```python
from build123d import *

# Parameters (mm, degrees)
SKETCH1_R               = 20
SKETCH1_R_2             = 5
BOSS_EXTRUDE1_DEPTH     = 166
ENL_V_START             = -142.6
ESQUISSE3_R             = 20
ESQUISSE3_R_2           = 17.5
ENL_V_MAT_EXTRU_1_DEPTH = 2.4
ENL_V_START_2           = -32.2
ESQUISSE4_R             = 20
ESQUISSE4_R_2           = 17.5
ENL_V_MAT_EXTRU_2_DEPTH = 2.4
BOSS_EXTRU_1_START      = -22.8
BOSS_EXTRU_1_DEPTH      = 12.6
ESQUISSE6_R             = 20
ESQUISSE6_R_2           = 5
BOSS_EXTRU_2_DEPTH      = 110
BOSS_EXTRU_3_START      = -132.8
ESQUISSE7_R             = 40
BOSS_EXTRU_3_DEPTH      = 6
BOSS_EXTRU_4_START      = -30.2
ESQUISSE8_R             = 30
BOSS_EXTRU_4_DEPTH      = 10
CONG_3_R                = 19
ECHELLE1_SCALE          = 0.25


with BuildPart() as part:
    # Sketch1 → Boss-Extrude1 (new body)
    with BuildSketch(Plane.XY):
        Circle(SKETCH1_R)
        Circle(SKETCH1_R_2, mode=Mode.SUBTRACT)
    extrude(amount=BOSS_EXTRUDE1_DEPTH)

    # Esquisse3 → Enlèv. mat.-Extru.1 (cut)
    with BuildSketch(Plane.XY.offset(166).offset(ENL_V_START)):
        Circle(ESQUISSE3_R)
        Circle(ESQUISSE3_R_2, mode=Mode.SUBTRACT)
    extrude(amount=ENL_V_MAT_EXTRU_1_DEPTH, mode=Mode.SUBTRACT)

    # Esquisse4 → Enlèv. mat.-Extru.2 (cut)
    with BuildSketch(Plane.XY.offset(166).offset(ENL_V_START_2)):
        Circle(ESQUISSE4_R)
        Circle(ESQUISSE4_R_2, mode=Mode.SUBTRACT)
    extrude(amount=ENL_V_MAT_EXTRU_2_DEPTH, mode=Mode.SUBTRACT)

    # Esquisse5 → Boss.-Extru.1 (add)
    with BuildSketch(Plane.XY.offset(166).offset(BOSS_EXTRU_1_START)):
        with BuildLine():
            Line((-19.364916731, 5), (-26.364916731, 5))
            ThreePointArc((-26.364916731, 5), (-31.364916731, 0), (-26.364916731, -5))
            Line((-26.364916731, -5), (-19.364916731, -5))
            ThreePointArc((-19.364916731, -5), (-20, 0), (-19.364916731, 5))
        make_face()
        with BuildLine():
            Line((19.364916731, -5), (26.364916731, -5))
            ThreePointArc((26.364916731, -5), (31.364916731, 0), (26.364916731, 5))
            Line((26.364916731, 5), (19.364916731, 5))
            ThreePointArc((19.364916731, 5), (20, 0), (19.364916731, -5))
        make_face()
    extrude(amount=BOSS_EXTRU_1_DEPTH)

    # Esquisse6 → Boss.-Extru.2 (add)
    with BuildSketch(Plane.XY.offset(166)):
        Circle(ESQUISSE6_R)
        Circle(ESQUISSE6_R_2, mode=Mode.SUBTRACT)
    extrude(amount=BOSS_EXTRU_2_DEPTH)

    # Esquisse7 → Boss.-Extru.3 (add)
    with BuildSketch(Plane.XY.offset(276).offset(BOSS_EXTRU_3_START)):
        Circle(ESQUISSE7_R)
    extrude(amount=-BOSS_EXTRU_3_DEPTH)

    # Esquisse8 → Boss.-Extru.4 (add)
    with BuildSketch(Plane.XY.offset(276).offset(BOSS_EXTRU_4_START)):
        Circle(ESQUISSE8_R)
    extrude(amount=BOSS_EXTRU_4_DEPTH)

    # Congé3
    # the kernel refuses this fillet: 19 mm, written as the material it takes off along each edge
    with BuildSketch(Plane(origin=(0, 0, 276), x_dir=(1, 0, 0), z_dir=(0, -1, 0))) as cong_3_piece_1:
        with BuildLine():
            CenterArc((1, -18.574175621), CONG_3_R, 0, 77.846802531)
            Line((5, 0), (5.08, 0.371483512))
            ThreePointArc((5.08, 0.371483512), (12.5, 0.38), (20, 0.38))
            Line((20, 0.38), (20.38, 0))
            Line((20.38, 0), (20.38, -18.574175621))
            Line((20.38, -18.574175621), (20, -18.574175621))
        make_face()
    revolve(axis=Axis((0, 0, 276), (0, 0, 1)), mode=Mode.SUBTRACT)


with BuildPart() as part_1:
    # Echelle1: scaled about (0, 0, 140.981437802)
    add(part.part.scale(ECHELLE1_SCALE).moved(Location((0, 0, 105.736078351))))


solid = part_1.part
```
The listing builds one solid part. Answer for the finished solid, in the listing's coordinates (mm). A direction names the side the tool comes from. Coordinates: 2 decimals unless noted, no trailing zeros. Write each loop counter-clockwise with the first axis right and the second up, starting at its lowest first coordinate (ties: lowest second). Pieces come first, ordered by that corner, then holes. Notation, with made-up numbers: (-18, 32.25) - (-14, 32.25) arc R29 ccw to (-14, 57.25) - close; hole circle Ø11 at (61.25, 88). An arc over 180 degrees is marked (long way). Return JSON: item names as keys, results as strings. Group by question number.
1. A cutting plane is placed at B-B, the plane z = 168.5. Determine the outline of the cut face in (x, y), plus the area to 3 significant figures.
2. A cutting plane is placed at A-A, the plane y = 6. Determine the outline of the cut face in (x, z), plus the area to 3 significant figures.
3. A cutting plane is placed at C-C, the plane z = 150.5. Determine the outline of the cut face in (x, y).
4. Given pin 1 (3 mm diameter, centred on y = 4, z = 122.5, fed in from -X); pin 2 (3 mm diameter, centred on x = 0, y = 0, fed in from +Z); pin 3 (1.2 mm diameter, centred on x = 0, y = -0.5, fed in from -Z); pin 4 (1.5 mm diameter, centred on y = 2, z = 161, fed in from -X), each flat-ended and moving along its own axis, determine where each tip first touches the part or whether it passes through.
5. Determine the mould class of faces 1 (the cylindrical face through (-7.84, 0.03, 143.09)), 2 (the flat face through (-5, -2, 140.036)), 3 (the flat face through (0, 0, 167.186)) for opening direction X: released by +X, released by -X, zero draft, split by the parting line, or undercut.
6. Straight lines are drawn through the part: L1, parallel to Z at x = -3.5, y = 5.75; L2, parallel to Z at x = -3.5, y = 8.25; L3, parallel to X at y = 0, z = 171.15. For each, find the intervals that lie inside material, in ascending order.
7. Which of the six approach directions +Z, -Z, +X, -X, +Y, -Y give full straight-line access (tool end or side, diameter ignored) to faces 4 (the flat face through (6, 1.25, 143)), 5 (the flat face through (-6, 1.25, 143)), 6 (the cylindrical face through (-7.493, 0.33, 168.419))?
Ans:
{
 "1": {"outline": "circle Ø15 at (0, 0)", "area": "177 mm²"},
 "2": {"outline": "(-8, 140.04) - (8, 140.04) - (8, 141.54) - (-8, 141.54) - close; (-4.5, 167.19) - (4.5, 167.19) - (4.5, 169.69) - (-4.5, 169.69) - close", "area": "46.5 mm²"},
 "3": {"outline": "circle Ø10 at (0, 0); hole circle Ø2.5 at (0, 0)"},
 "4": {"pin 1": "x = -4.33", "pin 2": "z = 174.74", "pin 3": "z = 140.04", "pin 4": "x = -4.84"},
 "5": {"face 1": "released by -X", "face 2": "zero draft", "face 3": "undercut"},
 "6": {"L1": "140.04 to 141.54, 167.19 to 169.69", "L2": "140.04 to 141.54", "L3": "-4.88 to -1.25, 1.25 to 4.88"},
 "7": {"face 4": "+X, +Y", "face 5": "-X, +Y", "face 6": "+Z"}
}
